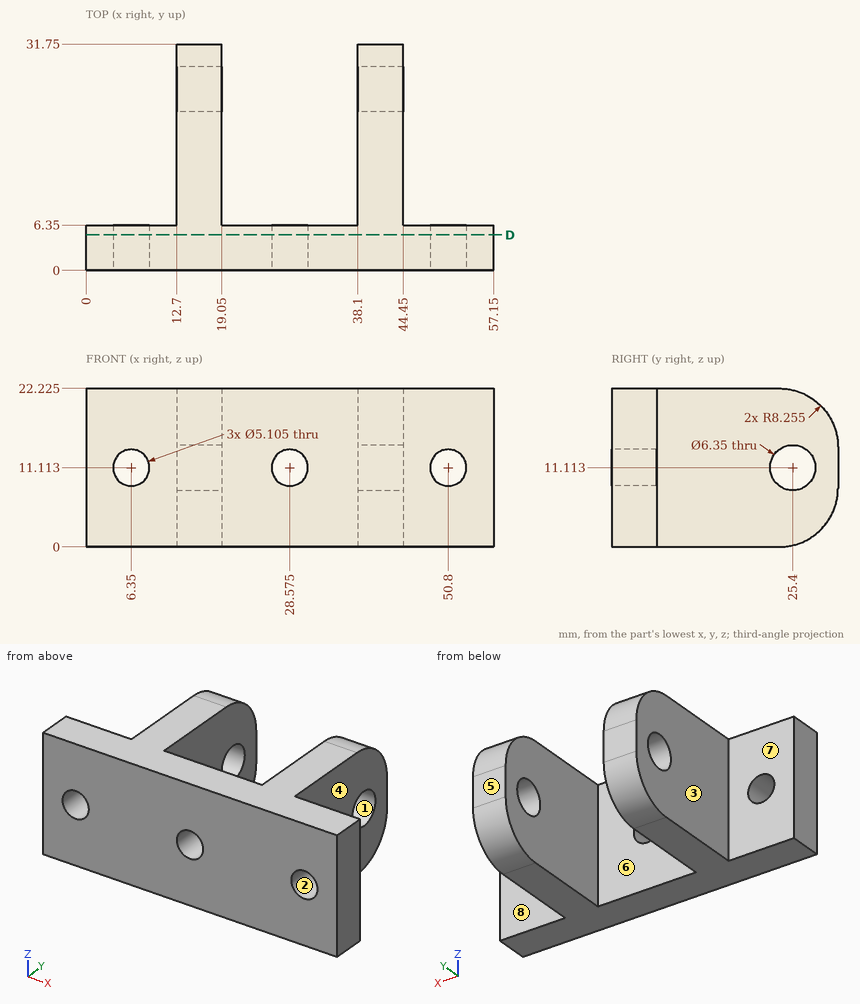
Verification items for this drawing (mm, ordinates from the low corner). A direction names the side the tool comes from. Round coordinates to 2 decimals unless told otherwise and drop trailing zeros.
1) Material ranges on line 1 (X direction, y = 22, z = 5.25); line 2 (Z direction, x = 50, y = 1) (1 decimal); line 3 (Y direction, x = 33, z = 13), recorded low to high.
Geometry says:
line 1: x = 12.7 to 19.05, 38.1 to 44.45
line 2: z = 0 to 8.7, 13.5 to 22.2
line 3: y = 0 to 6.35
2) Tool access check on the marked faces 5, 6, 7 and 8. Record the directions out of +Z, -Z, +X, -X, +Y, -Y that give a thin tool (end or side, any length) a straight path to the whole face; none if there is none.
Geometry says:
face 5: +Z, -Z, +X, -X, +Y
face 6: +Z, -Z, +Y
face 7: +Z, -Z, -X, +Y
face 8: +Z, -Z, +X, +Y
3) Depth check by flat-ended pin: pin 1 (6.5 mm diameter, centred on y = 15.5, z = 12, fed in from -X); pin 2 (3 mm diameter, centred on x = 35.5, y = 17, fed in from -Z); pin 3 (3 mm diameter, centred on y = 25.5, z = 5, fed in from +X); pin 4 (3 mm diameter, centred on x = 16, z = 2.5, fed in from +Y). Enter the tip coordinate at first touch or a pass-through.
Geometry says:
pin 1: stops at x = 12.7
pin 2: passes through
pin 3: stops at x = 44.45
pin 4: stops at y = 30.57
4) Cross-section at D-D, the plane y = 5. Give the number of separate pieces and of enclosed holes in the cut face, plus the area to 3 significant figures.
Geometry says:
separate pieces: 1
enclosed holes: 3
area: 1,210 mm2
5) Draft check along X on the marked faces 1, 2, 3 and 4. Enter one of: +X half, -X half, draft (parallel to the pull), parting line (faces both ways), or undercut.
Geometry says:
face 1: draft
face 2: undercut
face 3: -X half
face 4: +X half
